```python
from build123d import *

# Parameters (mm, degrees)
SKETCH_1_R          = 2.55
EXTRUDE_1_DEPTH     = 5
FILLET_1_R          = 10
CUT_EXTRUDE_1_DEPTH = 94.139680051


with BuildPart() as part:
    # ｽｹｯﾁ1 → ﾎﾞｽ - 押し出し1 (new body)
    with BuildSketch(Plane.XY):
        Polygon((0, -25), (0, 0), (-25, 0), (-25, 20), (0, 20), (35, 55), (35, 75), (55, 75), (55, 35), (20, 0), (20, -25), align=None)
        with Locations((-12.5, 10)):
            Circle(SKETCH_1_R, mode=Mode.SUBTRACT)
        with Locations((10, -12.5)):
            Circle(SKETCH_1_R, mode=Mode.SUBTRACT)
        with Locations((45, 65)):
            Circle(SKETCH_1_R, mode=Mode.SUBTRACT)
    extrude(amount=EXTRUDE_1_DEPTH)

    # ﾌｨﾚｯﾄ1
    fillet_1_edges = [part.edges().sort_by_distance(p)[0] for p in [
        (35, 75, 2.5),
        (55, 75, 2.5),
        (20, 0, 2.5),
        (20, -25, 2.5),
        (0, -25, 2.5),
        (0, 0, 2.5),
        (-25, 0, 2.5),
        (-25, 20, 2.5),
        (0, 20, 2.5),
        (35, 55, 2.5),
        (55, 35, 2.5),
    ]]
    fillet(fillet_1_edges, radius=FILLET_1_R - 0.0001)  # a hair under: the kernel refuses the full size

    # ｽｹｯﾁ2 → ｶｯﾄ - 押し出し1 (cut, through all)
    with BuildSketch(Plane.XY.offset(5)):
        with BuildLine():
            Line((4.393398282, 17.32233047), (34.393398282, 47.32233047))
            ThreePointArc((34.393398282, 47.32233047), (47.32233047, 47.32233047), (47.32233047, 34.393398282))
            Line((47.32233047, 34.393398282), (17.32233047, 4.393398282))
            ThreePointArc((17.32233047, 4.393398282), (4.393398282, 4.393398282), (4.393398282, 17.32233047))
        make_face()
    extrude(amount=-CUT_EXTRUDE_1_DEPTH, mode=Mode.SUBTRACT)


solid = part.part
```
Could you check a few things on this model? Use its own coordinates, in mm. A direction names the side the tool comes from. Coordinates: 2 decimals unless noted, no trailing zeros. Loops run counter-clockwise (first coordinate to the right, second up) from the corner with the lowest first, then second, coordinate; pieces in that order, holes last.
1) Please list where these lines run through material, in increasing order: line 1 along Y through (x, z) = (-12.5, 3.9); line 2 along Y through (x, z) = (11, 4.8); line 3 along Y through (x, z) = (10, 2.25).
Reported:
line 1: y = 0 to 7.45, 12.55 to 20
line 2: y = -24.95 to -14.85, -10.15 to 1.72, 23.93 to 31
line 3: y = -25 to -15.05, -9.95 to 1.76, 22.93 to 30
2) Which directions (+Z, -Z, +X, -X, +Y, -Y) give clear straight access to the entire face, cutting with the end or side of a thin tool? Please do faces 5 (the face through (15, 29, 5)), 6 (the face through (17, 37, 2)), 7 (the face through (32.53, 19.6, 2.54)), 8 (the face through (20, -9, 2)), 9 (the face through (-12, 0, 2)).
Reported:
face 5: +Z, +X, -X, +Y, -Y
face 6: +Z, -Z, -X, +Y
face 7: +Z, -Z
face 8: +Z, -Z, +X, -Y
face 9: +Z, -Z, -X, -Y
3) Imagine slicing it at A-A (y = -12.5). List the corners of the cut face in (x, z) for me.
Reported:
outline: (0, 0) - (7.45, 0) - (7.45, 5) - (0, 5) - close; (12.55, 0) - (20, 0) - (20, 5) - (12.55, 5) - close
4) Thinking about a two-plate mould opening in Y: for faces 1 (the face through (15, 29, 0)), 2 (the face through (47.18, 47.46, 2.54)), 3 (the face through (16.99, -22.15, 2.54)), 4 (the face through (43.1, 66.7, 2.5)), which applies, released by +Y, released by -Y, zero draft, split by the parting line, or undercut?
Reported:
face 1: zero draft
face 2: undercut
face 3: released by -Y
face 4: undercut
5) Imagine slicing it at B-B (z = 1.35). State how many separate pieces and enclosed holes the cut face has, and give its area (3 significant figures).
Reported:
separate pieces: 1
enclosed holes: 4
area: 2,000 mm2
6) Will these pins go through, and if not, where does the flat tip stop? pin 1 Ø3 at (y, z) = (48, 2.5) entering from -X; pin 2 Ø2.5 at (x, z) = (-10, 2.5) entering from +Y.
Reported:
pin 1: stops at x = 26.5
pin 2: stops at y = 20
